Geometry check sheet. Reference: drawing and pictorial views, mm from the part's lowest x, y, z. A direction names the side the tool comes from. Give positions to 0.01 mm unless a question says otherwise; leave off trailing zeros. Order: outer loops, then holes, each group sorted by start corner. A loop starts at its lowest first (then second) coordinate and runs counter-clockwise, first axis right, second up.
Item 1: Material ranges on line 1 along Y through (x, z) = (2.25, 1.75); line 2 along Y through (x, z) = (4.75, 1); line 3 along Z through (x, y) = (4.5, 1.75), recorded low to high.
Item 2: Access from +Z, -Z, +X, -X, +Y, -Y to the whole of each face (thin tool, end or side, straight path). Record for the marked faces 1 and 2.
Item 3: Sectioned sample at B-B on y = 13.75. Record the boundary of the cut face in (x, z).
Item 4: Sectioned sample at A-A on y = 8.5. Record the boundary of the cut face in (x, z), and give its area (3 significant figures).
Item 5: Gauge pin test, flat ends, axial feed: P1, Ø5, axis at y = 2, z = 7.5, coming from the +X side; P2, Ø1, axis at x = 3, z = 1.5, coming from the -Y side; P3, Ø6, axis at x = 1.5, y = 12, coming from the +Z side (3 decimals). Record the tip position at first contact, or that the pin passes through.
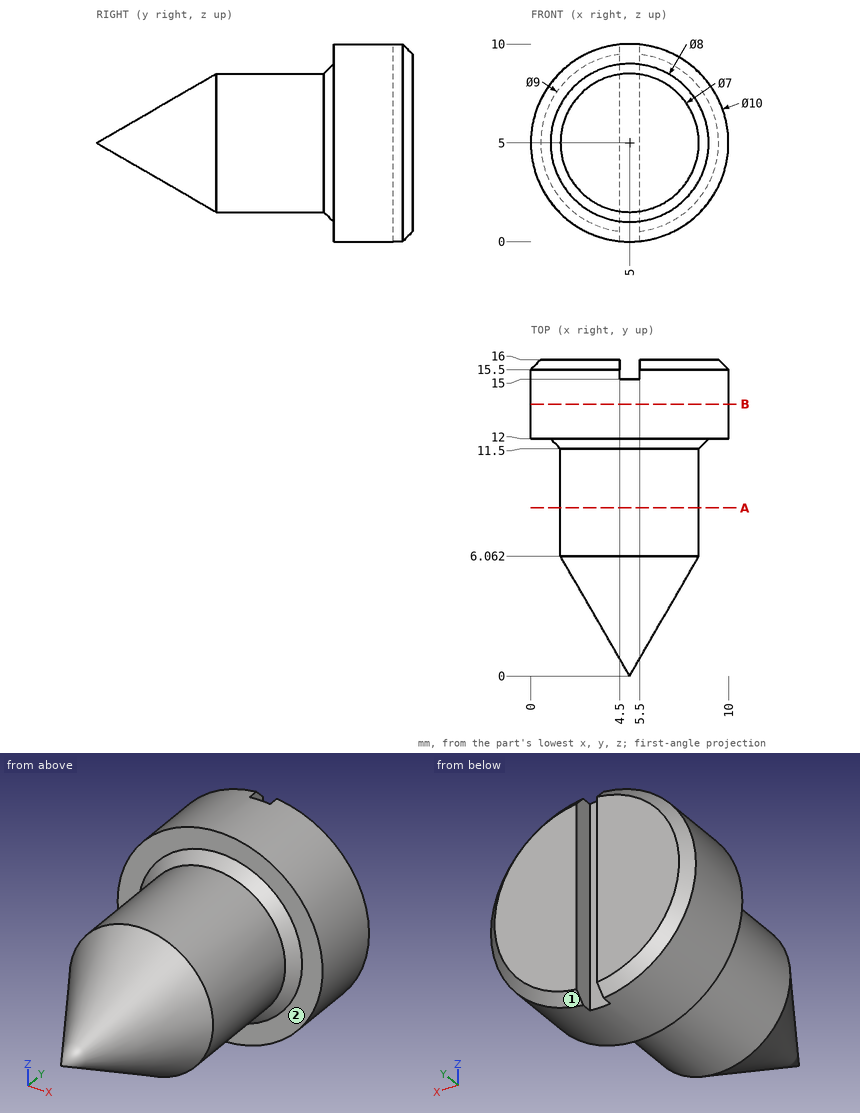
Report:
1. line 1: y = 12 to 16
1. line 2: y = 12 to 15
1. line 3: z = 4.12 to 5.88
2. face 1: +X, +Y
2. face 2: -Y
3. outline: circle Ø10 at (5, 5)
4. outline: circle Ø7 at (5, 5)
4. area: 38.5 mm2
5. P1: stops at x = 7.08
5. P2: stops at y = 11.53
5. P3: stops at z = 9.975
